```python
from build123d import *

# Parameters (mm, degrees)
F0_W     = 43
F0_H     = 38
F0_R     = 2
F0_R_2   = 7
F1_DEPTH = 4
F2_W     = 8.5
F2_H     = 6
F2_R     = 2
F3_DEPTH = 8
F4_W     = 3
F4_H     = 26
F5_DEPTH = 25
F6_R     = 2.99999
F7_R     = 0.7


# Not quite as in the source:
# - a fillet or chamfer is up to 0.001 mm smaller than in the source, because OpenCascade refuses the exact size


with BuildPart() as f1:
    # F0 (on Top) → F1 (new body)
    with BuildSketch(Plane.XY):
        Rectangle(F0_W, F0_H)
        with Locations((-16, -16)):
            Circle(F0_R, mode=Mode.SUBTRACT)
        with Locations((-8, -16)):
            Circle(F0_R, mode=Mode.SUBTRACT)
        with Locations((-16, -8)):
            Circle(F0_R, mode=Mode.SUBTRACT)
        with BuildLine():
            ThreePointArc((-9.4142135624, -6.5857864376), (-6.5857864376, -6.5857864376), (-6.5857864376, -9.4142135624))
            Line((-6.5857864376, -9.4142135624), (-7.0710678119, -9.8994949366))
            ThreePointArc((-7.0710678119, -9.8994949366), (-9.8994949366, -9.8994949366), (-9.8994949366, -7.0710678119))
            Line((-9.8994949366, -7.0710678119), (-9.4142135624, -6.5857864376))
        make_face(mode=Mode.SUBTRACT)
        with Locations((8, -16)):
            Circle(F0_R, mode=Mode.SUBTRACT)
        with Locations((0, -12)):
            Circle(F0_R, mode=Mode.SUBTRACT)
        with Locations((16, -16)):
            Circle(F0_R, mode=Mode.SUBTRACT)
        with BuildLine():
            ThreePointArc((6.5857864376, -9.4142135624), (6.5857864376, -6.5857864376), (9.4142135624, -6.5857864376))
            Line((9.4142135624, -6.5857864376), (9.8994949366, -7.0710678119))
            ThreePointArc((9.8994949366, -7.0710678119), (9.8994949366, -9.8994949366), (7.0710678119, -9.8994949366))
            Line((7.0710678119, -9.8994949366), (6.5857864376, -9.4142135624))
        make_face(mode=Mode.SUBTRACT)
        with Locations((16, -8)):
            Circle(F0_R, mode=Mode.SUBTRACT)
        with Locations((-12, 0)):
            Circle(F0_R, mode=Mode.SUBTRACT)
        with Locations((-16, 8)):
            Circle(F0_R, mode=Mode.SUBTRACT)
        with BuildLine():
            ThreePointArc((-6.5857864376, 9.4142135624), (-6.5857864376, 6.5857864376), (-9.4142135624, 6.5857864376))
            Line((-9.4142135624, 6.5857864376), (-9.8994949366, 7.0710678119))
            ThreePointArc((-9.8994949366, 7.0710678119), (-9.8994949366, 9.8994949366), (-7.0710678119, 9.8994949366))
            Line((-7.0710678119, 9.8994949366), (-6.5857864376, 9.4142135624))
        make_face(mode=Mode.SUBTRACT)
        with Locations((-16, 16)):
            Circle(F0_R, mode=Mode.SUBTRACT)
        with Locations((-8, 16)):
            Circle(F0_R, mode=Mode.SUBTRACT)
        Circle(F0_R_2, mode=Mode.SUBTRACT)
        with BuildLine():
            ThreePointArc((9.4142135624, 6.5857864376), (6.5857864376, 6.5857864376), (6.5857864376, 9.4142135624))
            Line((6.5857864376, 9.4142135624), (7.0710678119, 9.8994949366))
            ThreePointArc((7.0710678119, 9.8994949366), (9.8994949366, 9.8994949366), (9.8994949366, 7.0710678119))
            Line((9.8994949366, 7.0710678119), (9.4142135624, 6.5857864376))
        make_face(mode=Mode.SUBTRACT)
        with Locations((12, 0)):
            Circle(F0_R, mode=Mode.SUBTRACT)
        with Locations((16, 8)):
            Circle(F0_R, mode=Mode.SUBTRACT)
        with Locations((0, 12)):
            Circle(F0_R, mode=Mode.SUBTRACT)
        with Locations((8, 16)):
            Circle(F0_R, mode=Mode.SUBTRACT)
        with Locations((16, 16)):
            Circle(F0_R, mode=Mode.SUBTRACT)
    extrude(amount=F1_DEPTH)

    # F2 (on face) → F3 (join)
    with BuildSketch(Plane.XY.offset(4)):
        with Locations((-17.25, 16)):
            Rectangle(F2_W, F2_H)
        with Locations((-16, 16)):
            Circle(F2_R, mode=Mode.SUBTRACT)
        with Locations((17.25, 16)):
            Rectangle(F2_W, F2_H)
        with Locations((16, 16)):
            Circle(F2_R, mode=Mode.SUBTRACT)
        with Locations((17.25, -16)):
            Rectangle(F2_W, F2_H)
        with Locations((16, -16)):
            Circle(F2_R, mode=Mode.SUBTRACT)
        with Locations((-17.25, -16)):
            Rectangle(F2_W, F2_H)
        with Locations((-16, -16)):
            Circle(F2_R, mode=Mode.SUBTRACT)
    extrude(amount=F3_DEPTH)

    # F4 (on face) → F5 (cut)
    with BuildSketch(Plane.XY.offset(4)):
        with Locations((-20, 0)):
            Rectangle(F4_W, F4_H)
        with Locations((20, 0)):
            Rectangle(F4_W, F4_H)
    extrude(amount=-F5_DEPTH, mode=Mode.SUBTRACT)

    # F6 (radius 3 in the source; OpenCascade refuses exactly that, so slightly less here)
    f6_edges = [f1.edges().sort_by_distance(p)[0] for p in [
        (-18.5, 13, 2),
        (-18.5, -13, 2),
        (18.5, 13, 2),
        (18.5, -13, 2),
    ]]
    fillet(f6_edges, radius=F6_R)

    # F7
    f7_edges = [f1.edges().sort_by_distance(p)[0] for p in [
        (13, 13, 8),
        (13, -19, 8),
        (13, -13, 8),
        (-13, -19, 8),
        (-13, 13, 8),
        (-13, 19, 8),
        (-13, -13, 8),
        (13, 19, 8),
    ]]
    fillet(f7_edges, radius=F7_R)


solid = f1.part
```
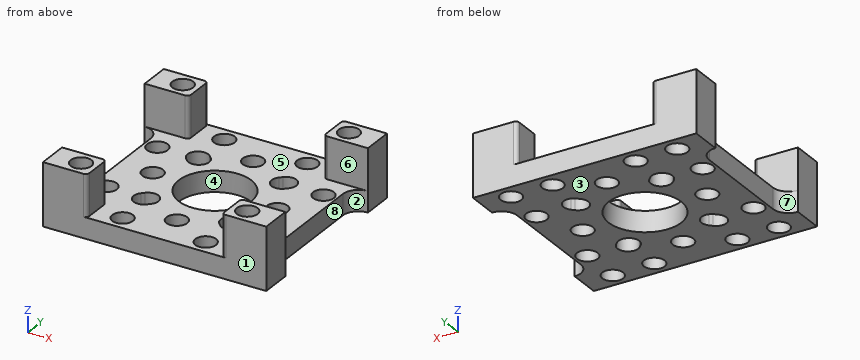
Input: part model. Units: mm. Frame: model coordinates. Face numbers are marked on the shaded views. A direction names the side the tool comes from. Round coordinates to 2 decimals unless told otherwise and drop trailing zeros. Loops run counter-clockwise (first coordinate to the right, second up) from the corner with the lowest first, then second, coordinate; pieces in that order, holes last. Notation, with made-up numbers: (83.25, -26) - (87.25, -26) arc R19 cw to (87.25, -8) - close; hole circle Ø6 at (-29, 43). An arc over 180 degrees is marked (long way). One line per item, written item: value. Start each with the question number.
(1) Section A-A, the plane z = 10. Return loops of the section in (x, y), plus the area to 3 significant figures.
(2) Access query for the marked faces 5, 6, 7 and 8. Directions: +Z, -Z, +X, -X, +Y, -Y. A direction counts if a zero-diameter tool reaches every point of the face in a straight line with its end or side. Return the directions, or none.
(3) Section B-B, the plane x = -12. Return loops of the section in (y, z), plus the area to 3 significant figures.
(4) Ray query, line 1 (Y direction, x = -16, z = 1.55); line 2 (Y direction, x = 15, z = 9); line 3 (X direction, y = -15, z = 10.5). Return the intervals inside material, ascending. Write a range as [from, to].
(5) Section C-C, the plane y = 16. Return loops of the section in (x, z), plus the area to 3 significant figures.
(6) Contact query for flat-ended pins moving along their axis: P1, Ø2, axis at y = 0.5, z = 2, coming from the -X side; P2, Ø10, axis at x = 4, y = 11.5, coming from the +Z side; P3, Ø2, axis at y = -0.5, z = 2.5, coming from the +X side; P4, Ø3.5, axis at x = 12, y = 0, coming from the +Z side. Output: stop coordinate, or through.
(7) Draft query along Y for the marked faces 1, 2, 3 and 4. Return one class per face: +Y half, -Y half, draft (parallel to the pull), parting line (faces both ways), or undercut.
(8) Section D-D, the plane y = 0. Return loops of the section in (x, z).
Results below:
1. outline: (-21.5, -19) - (-13.7, -19) arc R0.7 ccw to (-13, -18.3) - (-13, -13.7) arc R0.7 ccw to (-13.7, -13) - (-21.5, -13) - close; (-21.5, 13) - (-13.7, 13) arc R0.7 ccw to (-13, 13.7) - (-13, 18.3) arc R0.7 ccw to (-13.7, 19) - (-21.5, 19) - close; (13, -18.3) arc R0.7 ccw to (13.7, -19) - (21.5, -19) - (21.5, -13) - (13.7, -13) arc R0.7 ccw to (13, -13.7) - close; (13, 13.7) arc R0.7 ccw to (13.7, 13) - (21.5, 13) - (21.5, 19) - (13.7, 19) arc R0.7 ccw to (13, 18.3) - close; hole circle Ø4 at (-16, -16); hole circle Ø4 at (-16, 16); hole circle Ø4 at (16, -16); hole circle Ø4 at (16, 16)
1. area: 153 mm^2
2. face 5: +Z
2. face 6: +Z, +X, -X
2. face 7: +Z, -Z, -X
2. face 8: +Z, -Z, +X
3. outline: (-19, 0) - (-2, 0) - (-2, 4) - (-19, 4) - close; (2, 0) - (19, 0) - (19, 4) - (2, 4) - close
3. area: 136 mm^2
4. line 1: [-19, -18], [-14, -10], [-6, 6], [10, 14], [18, 19]
4. line 2: [-19, -17.73], [-14.27, -13], [13, 14.27], [17.73, 19]
4. line 3: [-21.5, -17.73], [-14.27, -13], [13, 14.27], [17.73, 21.5]
5. outline: (-21.5, 0) - (-18, 0) - (-18, 12) - (-21.5, 12) - close; (-14, 0) - (-10, 0) - (-10, 4) - (-13, 4) - (-13, 12) - (-14, 12) - close; (-6, 0) - (6, 0) - (6, 4) - (-6, 4) - close; (10, 0) - (14, 0) - (14, 12) - (13, 12) - (13, 4) - (10, 4) - close; (18, 0) - (21.5, 0) - (21.5, 12) - (18, 12) - close
5. area: 180 mm^2
6. P1: x = -18.5
6. P2: z = 4
6. P3: x = 18.5
6. P4: through
7. face 1: -Y half
7. face 2: undercut
7. face 3: draft
7. face 4: undercut
8. outline: (-18.5, 0) - (-14, 0) - (-14, 4) - (-18.5, 4) - close; (-10, 0) - (-7, 0) - (-7, 4) - (-10, 4) - close; (7, 0) - (10, 0) - (10, 4) - (7, 4) - close; (14, 0) - (18.5, 0) - (18.5, 4) - (14, 4) - close
